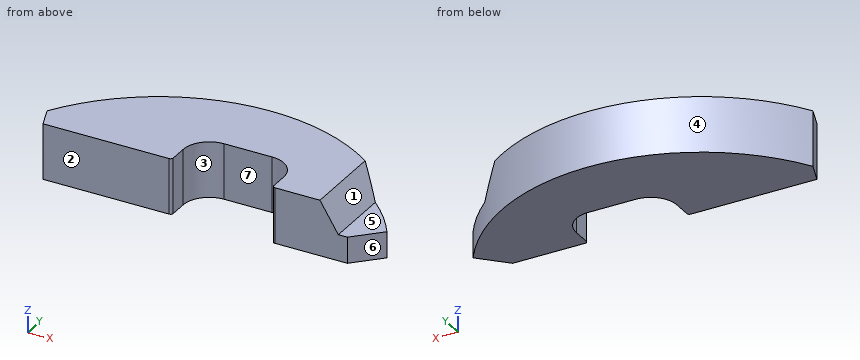
from build123d import *

# Parameters (mm, degrees)
BOSS_EXTRUDE1_DEPTH = 53.975
FILLET1_R           = 25.4
FILLET2_R           = 2.54
CHAMFER1_SIZE       = 38.1
CHAMFER2_SIZE       = 19.17726945
CUT_EXTRUDE2_DEPTH  = 221.930957303


with BuildPart() as part:
    # Sketch1 → Boss-Extrude1 (new body)
    with BuildSketch(Plane.XY):
        with BuildLine():
            Line((-48.768, 0), (-48.768, 45.106))
            Line((-48.768, 45.106), (48.768, 45.106))
            Line((48.768, 45.106), (48.768, 0))
            Line((48.768, 0), (159.817162922, 0))
            ThreePointArc((159.817162922, 0), (-16.571441881, 113.499698272), (-192.960046685, 0))
            Line((-192.960046685, 0), (-48.768, 0))
        make_face()
    extrude(amount=BOSS_EXTRUDE1_DEPTH)

    # Fillet1
    fillet1_edges = [part.edges().sort_by_distance(p)[0] for p in [
        (48.768, 45.106, 26.9875),
        (-48.768, 45.106, 26.9875),
    ]]
    fillet(fillet1_edges, radius=FILLET1_R)

    # Fillet2
    fillet2_edges = [part.edges().sort_by_distance(p)[0] for p in [
        (48.768, 0, 26.9875),
        (-48.768, 0, 26.9875),
    ]]
    fillet(fillet2_edges, radius=FILLET2_R)

    # Chamfer1
    # the kernel refuses this chamfer: 38.1, 28.765904175 mm, written as the material it takes off along each edge
    with BuildSketch(Plane(origin=(159.817162922, 0, -97.981121842), x_dir=(-0.47921828298651964, 0.8776957543770233, 0), z_dir=(0, 0, 1))) as chamfer1_piece_1:
        with BuildLine():
            Line((28.078418346, 0), (CHAMFER1_SIZE * 0.479218282987, CHAMFER1_SIZE * 0.877695754377))
            Line((CHAMFER1_SIZE * 0.479218282987, CHAMFER1_SIZE * 0.877695754377), (0, 0))
            ThreePointArc((0, 0), (14.253669202, -0.509031999), (28.078418346, 0))
        make_face()
    extrude(amount=249.937243683, mode=Mode.SUBTRACT)

    # Chamfer2
    # the kernel refuses this chamfer: 25.4, 19.17726945 mm, written as the material it takes off along each edge
    with BuildSketch(Plane(origin=(-192.960046685, 0, -61.621694141), x_dir=(1, 0, 0), z_dir=(0, 0, 1))) as chamfer2_piece_1:
        with BuildLine():
            Line((CHAMFER2_SIZE, 0), (11.259728132, 21.154322158))
            ThreePointArc((11.259728132, 21.154322158), (5.460860237, 11.048084579), (0, 0))
            Line((0, 0), (CHAMFER2_SIZE, 0))
        make_face()
    extrude(amount=177.218388283, mode=Mode.SUBTRACT)

    # Sketch2 → Cut-Extrude2 (cut, through all)
    with BuildSketch(Plane(origin=(0, 0, 0), x_dir=(1, 0, 0), z_dir=(0, 1, 0))):
        Polygon((112.968558119, -25.4), (49.468558119, -127), (163.768558119, -127), (163.768558119, -25.4), align=None)
    extrude(amount=CUT_EXTRUDE2_DEPTH, mode=Mode.SUBTRACT)


solid = part.part
CAD build for the part. Positions are in the model's coordinates, mm. Face numbers are marked on the shaded views. A direction names the side the tool comes from. Coordinates: 2 decimals unless noted, no trailing zeros. Loops run counter-clockwise (first coordinate to the right, second up) from the corner with the lowest first, then second, coordinate; pieces in that order, holes last. Notation, with made-up numbers: (-19.75, 60.5) - (25.25, 60.5) arc R25 cw to (25.25, 99.5) - close; hole circle Ø3 at (25, 58.5). An arc over 180 degrees is marked (long way). Use one line per item in the form item = value. Start each with the question number.
1) Band-saw the part on B-B (z = 13.5). Give the cut face in (x, y), and give its area (3 significant figures).
2) Drill centre lines: L1, parallel to X at y = 12, z = 50.5; L2, parallel to X at y = 38, z = 41.5; L3, parallel to Y at x = -105, z = 35.5. Where is each one in solid material? Low to high. Write a range as from..to.
3) Band-saw the part on A-A (y = 34.5). Give the cut face in (x, z) (3 decimals), and give its area (3 significant figures).
4) Band-saw the part on C-C (y = 9). Give the cut face in (x, z) (3 decimals).
5) Band-saw the part on D-D (x = -90). Give the cut face in (y, z) (3 decimals).
6) Two-plate mould, pull along X, no slides. Class the marked faces 1, 2, 3 and 4: +X half, -X half, draft (parallel to the pull), parting line (faces both ways), or undercut.
7) Flat gauge pins, fed straight in: pin 1 (1.5 mm diameter, centred on x = -83, z = 44.5, fed in from +Y); pin 2 (1 mm diameter, centred on y = 83.5, z = 25.5, fed in from -X); pin 3 (5 mm diameter, centred on x = -100.5, z = 6, fed in from +Y). Where does each tip first touch, or does it go through?
8) Tool access for the marked faces 5, 6 and 7: list every direction of +Z, -Z, +X, -X, +Y, -Y with a clear straight run to the whole face (end or side of a thin tool).
Check values:
q1.outline = (-181.7, 21.15) - (-173.78, 0) - (-51.31, 0) arc R2.54 ccw to (-48.77, 2.54) - (-48.77, 19.71) arc R25.4 cw to (-23.37, 45.11) - (23.37, 45.11) arc R25.4 cw to (48.77, 19.71) - (48.77, 2.54) arc R2.54 ccw to (51.31, 0) - (121.72, 0) - (146.36, 24.64) arc R193.81 ccw to start
q1.area = 24,000 mm2
q2.L1 = -178.27..-48.77, 48.77..97.28
q2.L2 = -170.08..-40.99, 40.99..102.91
q2.L3 = 0..92.15
q3.outline = (-172.716, 0) - (-44.015, 0) - (-44.015, 53.975) - (-172.716, 53.975) - close; (44.015, 0) - (139.573, 0) - (139.573, 25.4) - (112.969, 25.4) - (95.109, 53.975) - (44.015, 53.975) - close
q3.area = 11,100 mm2
q4.outline = (-177.151, 0) - (-48.768, 0) - (-48.768, 53.975) - (-177.151, 53.975) - close; (48.768, 0) - (130.717, 0) - (130.717, 25.4) - (112.969, 25.4) - (95.109, 53.975) - (48.768, 53.975) - close
q5.outline = (0, 0) - (99.051, 0) - (99.051, 53.975) - (0, 53.975) - close
q6.face_1 = +X half
q6.face_2 = draft
q6.face_3 = undercut
q6.face_4 = parting line
q7.pin_1 = 102.03
q7.pin_2 = -120.94
q7.pin_3 = 95.56
q8.face_5 = +Z, +X, +Y, -Y
q8.face_6 = +Z, -Z, +X, -Y
q8.face_7 = +Z, -Z, -Y
